Build history of the part. All positions in model axes, mm. A direction names the side the tool comes from. Round coordinates to 2 decimals unless told otherwise and drop trailing zeros. Order: outer loops, then holes, each group sorted by start corner. A loop starts at its lowest first (then second) coordinate and runs counter-clockwise, first axis right, second up. Notation, with made-up numbers: (-10.75, -9) -> (11.25, -9) arc R12 ccw to (11.25, 5) -> close; hole circle Ø8 at (2.5, 11.5). An arc over 180 degrees is marked (long way). Write item = value, one per line.
from build123d import *

# Parameters (mm, degrees)
SKETCH1_W           = 108.475208614
SKETCH1_H           = 90.5
BOSS_EXTRUDE1_DEPTH = 3.175
SKETCH2_W           = 6.85
SKETCH2_H           = 10.5
CUT_EXTRUDE1_DEPTH  = 93.588961798
LPATTERN1_COUNT     = 2
LPATTERN1_PITCH     = 60
SKETCH3_W           = 19.995208614
SKETCH3_H           = 15
CUT_EXTRUDE2_DEPTH  = 93.588961798
SKETCH4_W           = 6.85
SKETCH4_H           = 10.5
CUT_EXTRUDE3_DEPTH  = 93.588961798
SHORT_DEPTH         = 93.588961798


with BuildPart() as part:
    # Sketch1 → Boss-Extrude1 (new, symmetric)
    with BuildSketch(Plane(origin=(0, 0, 0), x_dir=(1, 0, 0), z_dir=(0, 1, 0))):
        with Locations((3, -27.25)):
            Rectangle(SKETCH1_W, SKETCH1_H)
        Polygon((-22.762395693, 0), (-27.381197846, 8), (-36.618802154, 8), (-41.237604307, 0), (-36.618802154, -8), (-27.381197846, -8), align=None, mode=Mode.SUBTRACT)
        Polygon((41.237604307, 0), (36.618802154, 8), (27.381197846, 8), (22.762395693, 0), (27.381197846, -8), (36.618802154, -8), align=None, mode=Mode.SUBTRACT)
    extrude(amount=BOSS_EXTRUDE1_DEPTH, both=True)

    # Sketch2 → Cut-Extrude1 (cut, through all)
    with BuildSketch(Plane(origin=(0, 3.175, 0), x_dir=(1, 0, 0), z_dir=(0, 1, 0))):
        with Locations((-16.337395693, 12.75)):
            Rectangle(SKETCH2_W, SKETCH2_H)
        with Locations((-16.337395693, -67.25)):
            Rectangle(SKETCH2_W, SKETCH2_H)
        with Locations((-16.337395693, -27.25)):
            Rectangle(SKETCH2_W, SKETCH2_H)
    cut_extrude1 = extrude(amount=-CUT_EXTRUDE1_DEPTH, mode=Mode.SUBTRACT)

    # LPattern1: Cut-Extrude1 ×2
    with Locations(*[(i * LPATTERN1_PITCH, 0, 0) for i in range(1, LPATTERN1_COUNT)]):
        add(cut_extrude1, mode=Mode.SUBTRACT)

    # Sketch3 → Cut-Extrude2 (cut, through all)
    with BuildSketch(Plane(origin=(0, 3.175, 0), x_dir=(1, 0, 0), z_dir=(0, 1, 0))):
        with Locations((12, 10.5)):
            Rectangle(SKETCH3_W, SKETCH3_H)
    extrude(amount=-CUT_EXTRUDE2_DEPTH, mode=Mode.SUBTRACT)

    # Sketch4 → Cut-Extrude3 (cut, through all)
    with BuildSketch(Plane(origin=(0, 3.175, 0), x_dir=(1, 0, 0), z_dir=(0, 1, 0))):
        with Locations((50.512604307, -64.25)):
            Rectangle(SKETCH4_W, SKETCH4_H)
        with Locations((50.512604307, -31.95)):
            Rectangle(SKETCH4_W, SKETCH4_H)
    extrude(amount=-CUT_EXTRUDE3_DEPTH, mode=Mode.SUBTRACT)

    # Sketch5 → Short (cut, through all)
    with BuildSketch(Plane(origin=(0, 3.175, 0), x_dir=(1, 0, 0), z_dir=(0, 1, 0))):
        Polygon((-51.237604307, -72.5), (57.237604307, -72.5), (57.237604307, -18), (47.087604307, -18), (47.087604307, -7.5), (40.237604307, -7.5), (40.237604307, -18), (-12.912395693, -18), (-12.912395693, -7.5), (-19.762395693, -7.5), (-19.762395693, -18), (-51.237604307, -18), align=None)
    extrude(amount=-SHORT_DEPTH, mode=Mode.SUBTRACT)


solid = part.part
Q1. Cut at A-A, the plane z = 14. List the corners of the cut face in (x, y) (3 decimals).
Check values:
outline = (-51.238, -3.175) -> (-19.762, -3.175) -> (-19.762, 3.175) -> (-51.238, 3.175) -> close; (-12.912, -3.175) -> (40.238, -3.175) -> (40.238, 3.175) -> (-12.912, 3.175) -> close; (47.088, -3.175) -> (57.238, -3.175) -> (57.238, 3.175) -> (47.088, 3.175) -> close
Q2. Cut at D-D, the plane z = 5. List the corners of the cut face in (x, y) (3 decimals).
Check values:
outline = (-51.238, -3.175) -> (-38.351, -3.175) -> (-38.351, 3.175) -> (-51.238, 3.175) -> close; (-25.649, -3.175) -> (25.649, -3.175) -> (25.649, 3.175) -> (-25.649, 3.175) -> close; (38.351, -3.175) -> (57.238, -3.175) -> (57.238, 3.175) -> (38.351, 3.175) -> close
Q3. Probe probe 1 along X at (y, z) = (-2.5, 0); probe 2 along X at (y, z) = (2, -16); probe 3 along X at (y, z) = (2, 16). List the from-to ranges inside material, lowest first.
Check values:
probe_1 = -51.24 to -41.24, -22.76 to 22.76, 41.24 to 57.24
probe_2 = -51.24 to -19.76, -12.91 to 2, 22 to 40.24, 47.09 to 57.24
probe_3 = -51.24 to -19.76, -12.91 to 40.24, 47.09 to 57.24
Q4. Which spindle directions (+Z, -Z, +X, -X, +Y, -Y) get a long thin tool onto all of the face, cutting with end or side? Do faces 4 (the face through (-25.039, 0.044, -3.944)), 5 (the face through (-12.912, 0, -13)), 6 (the face through (-19.762, 0, 13)), 7 (the face through (-6, 0, -18)). Say none if no direction does.
Check values:
face_4 = +Y, -Y
face_5 = -Z, +Y, -Y
face_6 = +Z, +Y, -Y
face_7 = -Z, +X, -X, +Y, -Y
Q5. Cut at B-B, the plane x = 43.5. List the corners of the cut face in (y, z) (3 decimals), and give its area (4 significant figures).
Check values:
outline = (-3.175, -7.5) -> (3.175, -7.5) -> (3.175, 7.5) -> (-3.175, 7.5) -> close
area = 95.25 mm²
Q6. Cut at C-C, the plane y = -0.5. Give the number of separate pieces and of enclosed holes in the cut face, and give its area (3 significant figures).
Check values:
separate_pieces = 1
enclosed_holes = 2
area = 2,870 mm²
Q7. Flat gauge pins, fed straight in: pin 1 (1 mm diameter, centred on x = 45, y = 1, fed in from +Z); pin 2 (1.9 mm diameter, centred on x = -15.5, y = 0, fed in from -Z). Where does each tip first touch, or does it go through?
Check values:
pin_1 = 7.5
pin_2 = -7.5
Q8. Mould opens along X. For faces 1 (the face through (2, 3.175, 0)), 2 (the face through (44, 0, -7.5)), 3 (the face through (57.238, 0, 0)) say: released by +X, released by -X, zero draft, split by the parting line, or undercut.
Check values:
face_1 = zero draft
face_2 = undercut
face_3 = released by +X
